from build123d import *

# Parameters (mm, degrees)
SKETCH1_R           = 9.1
BOSS_EXTRUDE1_DEPTH = 6


with BuildPart() as part:
    # Sketch1 → Boss-Extrude1 (new body)
    with BuildSketch(Plane(origin=(0, 0, 0), x_dir=(0, 0, -1), z_dir=(1, 0, 0))):
        Polygon((-15, -25), (-15, 25), (-11.3, 25), (-11.3, 31), (-5.3, 31), (-5.3, 25), (-1.6, 25), (-1.6, 22), (-2.9, 22), (-2.9, 18.8), (-1.6, 18.8), (-1.6, 13), (1.6, 13), (1.6, 18.8), (2.9, 18.8), (2.9, 22), (1.6, 22), (1.6, 25), (5.3, 25), (5.3, 31), (11.3, 31), (11.3, 25), (15, 25), (15, -25), (11.3, -25), (11.3, -31), (5.3, -31), (5.3, -25), (1.6, -25), (1.6, -22), (2.9, -22), (2.9, -18.8), (1.6, -18.8), (1.6, -13), (-1.6, -13), (-1.6, -18.8), (-2.9, -18.8), (-2.9, -22), (-1.6, -22), (-1.6, -25), (-5.3, -25), (-5.3, -31), (-11.3, -31), (-11.3, -25), align=None)
        Circle(SKETCH1_R, mode=Mode.SUBTRACT)
    extrude(amount=BOSS_EXTRUDE1_DEPTH)


solid = part.part
Work out the finished part from the listing and answer in its coordinate system (mm). A direction names the side the tool comes from. Round coordinates to 2 decimals unless told otherwise and drop trailing zeros. Write each loop counter-clockwise with the first axis right and the second up, starting at its lowest first coordinate (ties: lowest second). Pieces come first, ordered by that corner, then holes.
1) A tool of negligible diameter and unlimited length cuts with its end or side. For faces 1 (the flat face through (3, 28, 5.3)), 2 (the flat face through (3, 25, -13)), 3 (the flat face through (3, -20, 2.9)), 4 (the flat face through (3, -16, -1.6)), from which of +Z, -Z, +X, -X, +Y, -Y can it reach the whole face along a straight path? Write none if from no direction.
2) Straight lines are drawn through the part: line 1 (Y direction, x = 4.05, z = 0); line 2 (Z direction, x = 4.05, y = 29.5); line 3 (Z direction, x = 5.75, y = 14). For each, find the intervals that lie inside material, in ascending order.
3) The mould has two halves that part along Y. Classify faces 5 (the flat face through (3, 25, 13)), 6 (the flat face through (3, 20, 2.9)), 7 (the flat face through (3, -23, 1.6)): pulls with the +Y half, pulls with the -Y half, needs draft (parallel to the pull), parting line crosses it, or undercut.
4) A cutting plane is placed at C-C (z = -12). Give the vertices of the cut face in (x, y), plus the area to 3 significant figures.
5) A cutting plane is placed at B-B (z = 0). Give the vertices of the cut face in (x, y), plus the area to 3 significant figures.
6) A cutting plane is placed at A-A (y = 23.5). Give the vertices of the cut face in (x, z), plus the area to 3 significant figures.
7) Given pin 1 Ø1.8 at (x, z) = (4.5, -2.5) entering from -Y; pin 2 Ø0.6 at (x, z) = (3.5, 2.5) entering from +Y; pin 3 Ø1.8 at (x, y) = (2.5, 27) entering from -Z; pin 4 Ø3 at (y, z) = (7, -0.5) entering from -X, each flat-ended and moving along its own axis, determine where each tip first touches the part or whether it passes through.
Completed:
1. face 1: +X, -X, +Y
1. face 2: -Z, +X, -X, +Y
1. face 3: +X, -X
1. face 4: +X, -X, -Y
2. line 1: y = -13 to -9.1, 9.1 to 13
2. line 2: z = -11.3 to -5.3, 5.3 to 11.3
2. line 3: z = -15 to -1.6, 1.6 to 15
3. face 5: pulls with the +Y half
3. face 6: undercut
3. face 7: needs draft
4. outline: (0, -25) - (6, -25) - (6, 25) - (0, 25) - close
4. area: 300 mm2
5. outline: (0, -13) - (6, -13) - (6, -9.1) - (0, -9.1) - close; (0, 9.1) - (6, 9.1) - (6, 13) - (0, 13) - close
5. area: 46.8 mm2
6. outline: (0, -15) - (6, -15) - (6, -1.6) - (0, -1.6) - close; (0, 1.6) - (6, 1.6) - (6, 15) - (0, 15) - close
6. area: 161 mm2
7. pin 1: stops at y = -25
7. pin 2: stops at y = 25
7. pin 3: stops at z = -11.3
7. pin 4: passes through
